Check sheet for the modelled part. Datum: model origin and axes. Units: mm. A direction names the side the tool comes from. Give positions to 0.01 mm unless a question says otherwise; leave off trailing zeros. Order: outer loops, then holes, each group sorted by start corner. A loop starts at its lowest first (then second) coordinate and runs counter-clockwise, first axis right, second up.
```python
from build123d import *

# Parameters (mm, degrees)
F1_DEPTH = 0.6
F2_DEPTH = 25
F3_W     = 0.8
F3_H     = 40
F7_DEPTH = 2


with BuildPart() as f1:
    # F0 (on Front) → F1 (new body)
    with BuildSketch(Plane.XZ):
        Polygon((0, -20), (0, 20), (-5, 15), (-5, -15), align=None)
        Polygon((-5, 15), (0, 20), (0, 21.1313708499), (-5.8, 15.3313708499), (-5.8, -15.3313708499), (0, -21.1313708499), (0, -20), (-5, -15), align=None)
    extrude(amount=-F1_DEPTH)

    # F0 (on Front) → F2 (join)
    with BuildSketch(Plane.XZ):
        Polygon((-5, 15), (0, 20), (0, 21.1313708499), (-5.8, 15.3313708499), (-5.8, -15.3313708499), (0, -21.1313708499), (0, -20), (-5, -15), align=None)
    extrude(amount=-F2_DEPTH)

    # F3 (on face) → F4 (join, up to the next surface of F1)
    with BuildSketch(Plane.YZ):
        with Locations((24.6, 0)):
            Rectangle(F3_W, F3_H)
        with BuildLine():
            ThreePointArc((8.2, -20), (16.4, 0), (8.2, 20))
            Line((8.2, 20), (7.6, 20))
            ThreePointArc((7.6, 20), (15.8, 0), (7.6, -20))
            Line((7.6, -20), (8.2, -20))
        make_face()
    extrude(until=Until.NEXT, dir=(-1, 0, 0))

    # F5: F1 across face


with BuildPart() as f1_1:
    add(f1.part)
    add(f1.part.mirror(Plane(origin=(0, 13.3750956502, 0), x_dir=(0, 1, 0), z_dir=(1, 0, 0))))

    # F6 (on face) → F7 (cut)
    with BuildSketch(Plane(origin=(0, 25, 0), x_dir=(-1, 0, 0), z_dir=(0, 1, 0))):
        with BuildLine():
            ThreePointArc((2.65, 8.5), (-1.8738329701, 10.3738329701), (0, 5.85))
            ThreePointArc((0, 5.85), (1.8738329701, 6.6261670299), (2.65, 8.5))
        make_face()
        with BuildLine():
            ThreePointArc((2.65, -8.5), (1.8738329701, -6.6261670299), (0, -5.85))
            ThreePointArc((0, -5.85), (-1.8738329701, -10.3738329701), (2.65, -8.5))
        make_face()
    extrude(amount=-F7_DEPTH, mode=Mode.SUBTRACT)


solid = f1_1.part
```
(1) Cross-section at A-A on x = 1.75. Enter the section's corners in (y, z).
Response values:
outline: (0, -19.38) - (25, -19.38) - (25, -10.49) - (24.2, -10.49) - (24.2, -18.25) - (9.79, -18.25) arc R28.49 ccw to (9.79, 18.25) - (24.2, 18.25) - (24.2, 10.49) - (25, 10.49) - (25, 19.38) - (0, 19.38) - close; (24.2, -6.51) - (25, -6.51) - (25, 6.51) - (24.2, 6.51) - close; hole (0.6, -18.25) - (9.19, -18.25) arc R28.49 ccw to (9.19, 18.25) - (0.6, 18.25) - close
(2) Cross-section at B-B on y = 5.5. Enter the section's corners in (x, z).
Response values:
outline: (-5.8, -15.33) - (0, -21.13) - (5.8, -15.33) - (5.8, 15.33) - (0, 21.13) - (-5.8, 15.33) - close; hole (-5, -15) - (0, -20) - (5, -15) - (5, 15) - (0, 20) - (-5, 15) - close
(3) Material ranges on L1, parallel to X at y = 24.45, z = 8.5; L2, parallel to Z at x = -4, y = 12.75; L3, parallel to X at y = 11, z = -7, recorded low to high.
Response values:
L1: x = -5.8 to -2.65, 2.65 to 5.8
L2: z = -17.13 to -16, -13.95 to -12.83, 12.83 to 13.95, 16 to 17.13
L3: x = -5.8 to -5, 5 to 5.8
(4) Release check for a two-part mould opening along Z. For faces 3 (the face through (0, 24.2, 0)), 4 (the face through (2.86, 12.32, 18.27)), 5 (the face through (2.94, 12.32, -18.19)) record: released by +Z, released by -Z, zero draft, split by the parting line, or undercut.
Response values:
face 3: undercut
face 4: released by +Z
face 5: released by -Z
(5) Cross-section at C-C on z = 6.5. Enter the section's corners in (x, y), then the cut area to 3 significant figures.
Response values:
outline: (-5.8, 0) - (5.8, 0) - (5.8, 25) - (1.74, 25) - (1.74, 24.2) - (5, 24.2) - (5, 15.65) - (-5, 15.65) - (-5, 24.2) - (-1.74, 24.2) - (-1.74, 25) - (-5.8, 25) - close; hole (-5, 0.6) - (5, 0.6) - (5, 15.05) - (-5, 15.05) - close
area: 57.2 mm2
(6) Set-up check for faces 1 (the face through (-2.94, 12.32, -18.19)), 2 (the face through (-3, 5, 17)): record each of +Z, -Z, +X, -X, +Y, -Y from which the full face is reachable in a straight line by a thin tool's end or side.
Response values:
face 1: -Z, -X, +Y, -Y
face 2: none
(7) Cross-section at D-D on y = 10. Enter the section's corners in (x, z), then the cut area to 3 significant figures.
Response values:
outline: (-5.8, -15.33) - (0, -21.13) - (5.8, -15.33) - (5.8, 15.33) - (0, 21.13) - (-5.8, 15.33) - close; hole (-5, -15) - (-2.77, -17.23) - (2.77, -17.23) - (5, -15) - (5, 15) - (2.77, 17.23) - (-2.77, 17.23) - (-5, 15) - close; hole (-2.01, -17.99) - (0, -20) - (2.01, -17.99) - close; hole (-2.01, 17.99) - (2.01, 17.99) - (0, 20) - close
area: 80.3 mm2
(8) Gauge pin test, flat ends, axial feed: pin 1 Ø1.5 at (x, y) = (2, 11.5) entering from -Z; pin 2 Ø3 at (x, z) = (0, 8.5) entering from +Y; pin 3 Ø5 at (x, y) = (-3.5, 21.5) entering from -Z. Record the tip position at first contact, or that the pin passes through.
Response values:
pin 1: stops at z = -19.88
pin 2: stops at y = 15.53
pin 3: stops at z = -20.13
